```python
from build123d import *

# Parameters (mm, degrees)
MODEL_W                 = 3
MODEL_H                 = 3
SALIENTE_EXTRUIR1_DEPTH = 1.5


with BuildPart() as part:
    # Model → Saliente-Extruir1 (new body)
    with BuildSketch(Plane.XY):
        with BuildLine():
            Line((9.904781567, 296.774995526), (99.904781567, 296.774995526))
            ThreePointArc((99.904781567, 296.774995526), (104.404781567, 292.274995526), (99.904781567, 287.774995526))
            Line((99.904781567, 287.774995526), (9.904781567, 287.774995526))
            ThreePointArc((9.904781567, 287.774995526), (5.404781567, 292.274995526), (9.904781567, 296.774995526))
        make_face()
        with Locations((9.904781567, 292.274995526)):
            Rectangle(MODEL_W, MODEL_H, mode=Mode.SUBTRACT)
        with Locations((18.904781567, 292.274995526)):
            Rectangle(MODEL_W, MODEL_H, mode=Mode.SUBTRACT)
        with Locations((27.904781567, 292.274995526)):
            Rectangle(MODEL_W, MODEL_H, mode=Mode.SUBTRACT)
        with Locations((36.904781567, 292.274995526)):
            Rectangle(MODEL_W, MODEL_H, mode=Mode.SUBTRACT)
        with Locations((45.904781567, 292.274995526)):
            Rectangle(MODEL_W, MODEL_H, mode=Mode.SUBTRACT)
        with Locations((54.904781567, 292.274995526)):
            Rectangle(MODEL_W, MODEL_H, mode=Mode.SUBTRACT)
        with Locations((63.904781567, 292.274995526)):
            Rectangle(MODEL_W, MODEL_H, mode=Mode.SUBTRACT)
        with Locations((72.904781567, 292.274995526)):
            Rectangle(MODEL_W, MODEL_H, mode=Mode.SUBTRACT)
        with Locations((81.904781567, 292.274995526)):
            Rectangle(MODEL_W, MODEL_H, mode=Mode.SUBTRACT)
        with Locations((90.904781567, 292.274995526)):
            Rectangle(MODEL_W, MODEL_H, mode=Mode.SUBTRACT)
        with Locations((99.904781567, 292.274995526)):
            Rectangle(MODEL_W, MODEL_H, mode=Mode.SUBTRACT)
    extrude(amount=SALIENTE_EXTRUIR1_DEPTH)


solid = part.part
```
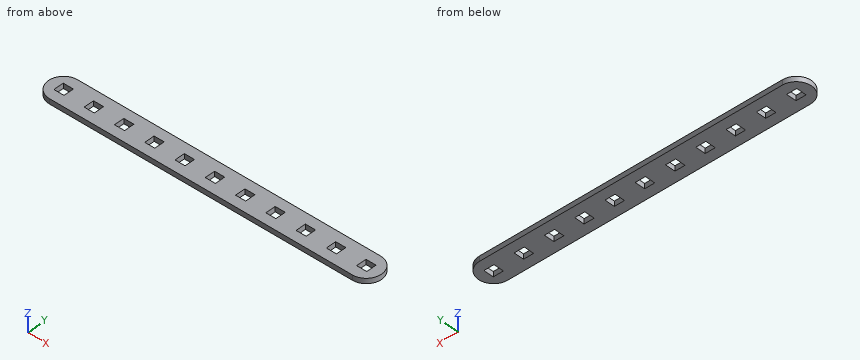
CAD build for the part. Positions are in the model's coordinates, mm. Give positions to 0.01 mm unless a question says otherwise; leave off trailing zeros. Loops run counter-clockwise (first coordinate to the right, second up) from the corner with the lowest first, then second, coordinate; pieces in that order, holes last. Notation, with made-up numbers: (-4, -27) -> (46, -27) arc R36 ccw to (46, 12) -> close; hole circle Ø2 at (59, -19.5). An arc over 180 degrees is marked (long way). Use a Markdown table: item, result.
1. Wall check: L1, parallel to Y at x = 46, z = 0.45 (3 decimals); L2, parallel to X at y = 290, z = 1.2; L3, parallel to X at y = 295.25, z = 0.1. Give the ranges that are in metal, low to high. Write a range as [from, to].
Check result:
| item | result |
|---|---|
| L1 | y = [287.775, 290.775], [293.775, 296.775] |
| L2 | x = [6.02, 103.79] |
| L3 | x = [6.53, 103.28] |
2. Slice it at D-D (y = 295.5). List the corners of the cut face in (x, z), plus the area to 3 significant figures.
Check result:
| item | result |
|---|---|
| outline | (6.77, 0) -> (103.04, 0) -> (103.04, 1.5) -> (6.77, 1.5) -> close |
| area | 144 mm^2 |
3. Slice it at B-B (z = 1). Give the number of separate pieces and of enclosed holes in the cut face, plus the area to 3 significant figures.
Check result:
| item | result |
|---|---|
| separate pieces | 1 |
| enclosed holes | 11 |
| area | 775 mm^2 |
4. Slice it at A-A (x = 18.5). List the corners of the cut face in (y, z) (3 decimals), plus the area to 3 significant figures.
Check result:
| item | result |
|---|---|
| outline | (287.775, 0) -> (290.775, 0) -> (290.775, 1.5) -> (287.775, 1.5) -> close; (293.775, 0) -> (296.775, 0) -> (296.775, 1.5) -> (293.775, 1.5) -> close |
| area | 9.00 mm^2 |
